```python
from build123d import *

# Parameters (mm, degrees)
F0_W     = 13.2459662855
F0_H     = 82.9233899713
F1_DEPTH = 74.4
F2_W     = 42.6411293447
F2_H     = 25.7661305368
F2_W_2   = 46.6330666095
F2_H_2   = 32.1169355884
F2_H_3   = 1.9959695637
F3_DEPTH = 25
F4_W     = 29.9395192415
F4_H     = 32.2983870283
F4_H_2   = 4.173386842
F4_H_3   = 25.040323846
F5_DEPTH = 10
F6_R     = 3.9795460227
F7_DEPTH = 90.9
F8_R     = 3.3126964472
F9_DEPTH = 59.4


with BuildPart() as f1:
    # F0 (on Front) → F1 (new body)
    with BuildSketch(Plane.XZ):
        with Locations((-51.7137106508, 3.0846782029)):
            Rectangle(F0_W, F0_H)
    extrude(amount=F1_DEPTH)

    # F2 (on face) → F3 (cut)
    with BuildSketch(Plane(origin=(-58.3366937935, 0, 0), x_dir=(0, -1, 0), z_dir=(-1, 0, 0))):
        with Locations((37.9233863205, 31.6633079201)):
            Rectangle(F2_W, F2_H)
        with Locations((36.1088728532, -22.3185489886)):
            Rectangle(F2_W_2, F2_H_2)
        with Locations((37.9233863205, 45.5443579704)):
            Rectangle(F2_W, F2_H_3)
    extrude(amount=-F3_DEPTH, mode=Mode.SUBTRACT)

    # F4 (on face) → F5 (cut)
    with BuildSketch(Plane(origin=(-58.3366937935, 0, 0), x_dir=(0, -1, 0), z_dir=(-1, 0, 0))):
        with Locations((36.4717757329, -22.4092747085)):
            Rectangle(F4_W, F4_H)
        with Locations((36.4717757329, 20.8669360727)):
            Rectangle(F4_W, F4_H_2)
        with Locations((36.4717757329, 6.2600807287)):
            Rectangle(F4_W, F4_H_3)
    extrude(amount=-F5_DEPTH, mode=Mode.SUBTRACT)

    # F6 (on face) → F7 (cut)
    with BuildSketch(Plane.XZ.offset(74.4)):
        with Locations((-52.8931468725, 19.3245988339)):
            Circle(F6_R)
    extrude(amount=-F7_DEPTH, mode=Mode.SUBTRACT)

    # F8 (on face) → F9 (cut)
    with BuildSketch(Plane(origin=(-48.3366937935, 0, 0), x_dir=(0, -1, 0), z_dir=(-1, 0, 0))):
        with Locations((33.8408090174, 7.0165661164)):
            Circle(F8_R)
    extrude(amount=-F9_DEPTH, mode=Mode.SUBTRACT)


solid = f1.part
```
Verification items for the finished model (mm, model axes). A direction names the side the tool comes from. Round coordinates to 2 decimals unless told otherwise and drop trailing zeros. Loops run counter-clockwise (first coordinate to the right, second up) from the corner with the lowest first, then second, coordinate; pieces in that order, holes last. Notation, with made-up numbers: (23.5, 84.25) -> (67.5, 84.25) arc R21 cw to (67.5, 111.25) -> close; hole circle Ø2 at (62.5, -30.75). An arc over 180 degrees is marked (long way). Answer as a JSON object with one key per item and string values.
Q1. Scan lines: line 1 (Y direction, x = -52, z = -28.5); line 2 (Y direction, x = -57.5, z = 25); line 3 (Z direction, x = -47.5, y = -23.5). Record each from-to range of solid material in increasing order. Write a range as from..to.
Data:
{"line 1": "y = -74.4..-59.43, -12.79..0", "line 2": "y = -74.4..-59.24, -16.6..0", "line 3": "z = -6.26..18.78"}
Q2. Access from +Z, -Z, +X, -X, +Y, -Y to the whole of each face (thin tool, end or side, straight path). Record for faces 1 (the flat face through (-52, -74.4, 4)), 2 (the flat face through (-52, -16.603, 32)), 3 (the flat face through (-53, -21.502, 6)), 4 (the flat face through (-52, -12.792, -23)).
Data:
{"face 1": "+Z, -Z, +X, -X, -Y", "face 2": "+Z, +X, -X", "face 3": "+Z, -Z, -X", "face 4": "-Z, +X, -X"}
Q3. Section check B-B (x = -53.25). Record the boundary of the cut face in (y, z).
Data:
{"outline": "(-74.4, -38.38) -> (-59.43, -38.38) -> (-59.43, -6.26) -> (-51.44, -6.26) -> (-51.44, 15.36) -> (-74.4, 15.36) -> close; (-74.4, 23.29) -> (-59.24, 23.29) -> (-59.24, 44.55) -> (-74.4, 44.55) -> close; (-21.5, -6.26) -> (-12.79, -6.26) -> (-12.79, -38.38) -> (0, -38.38) -> (0, 15.36) -> (-21.5, 15.36) -> close; (-16.6, 23.29) -> (0, 23.29) -> (0, 44.55) -> (-16.6, 44.55) -> close"}
Q4. Go/stop test with flat-tipped pins: P1, Ø12.5, axis at y = -34.5, z = 4, coming from the -X side; P2, Ø1.7, axis at x = -57.5, y = -18, coming from the +Z side. Record where each tip stops, or that it passes through.
Data:
{"P1": "stops at x = -48.34", "P2": "stops at z = 18.78"}
Q5. Draft check along Z on faces 5 (the flat face through (-47, -38, 18.78)), 6 (the cylindrical face through (-51.057, -10.902, 15.794)), 7 (the flat face through (-52, -67, -38.377)). Enter one of: pulls with the +Z half, pulls with the -Z half, needs draft (parallel to the pull), parting line crosses it, or undercut.
Data:
{"face 5": "pulls with the +Z half", "face 6": "undercut", "face 7": "pulls with the -Z half"}
Q6. Section check C-C (z = -1). Record the boundary of the cut face in (x, y).
Data:
{"outline": "(-58.34, -74.4) -> (-45.09, -74.4) -> (-45.09, 0) -> (-58.34, 0) -> (-58.34, -21.5) -> (-48.34, -21.5) -> (-48.34, -51.44) -> (-58.34, -51.44) -> close"}
Q7. Section check D-D (y = -61.5). Record the boundary of the cut face in (x, z), then the cut area to 3 significant figures.
Data:
{"outline": "(-58.34, -38.38) -> (-45.09, -38.38) -> (-45.09, 44.55) -> (-58.34, 44.55) -> close; hole circle Ø7.96 at (-52.89, 19.32)", "area": "1,050 mm2"}
Q8. Section check A-A (z = 35). Record the boundary of the cut face in (x, y).
Data:
{"outline": "(-58.34, -74.4) -> (-45.09, -74.4) -> (-45.09, -59.24) -> (-58.34, -59.24) -> close; (-58.34, -16.6) -> (-45.09, -16.6) -> (-45.09, 0) -> (-58.34, 0) -> close"}
